from build123d import *

# Parameters (mm, degrees)
F0_R     = 49.7765250683
F1_DEPTH = 152.4
F2_R     = 25.4
F4_D     = 76.2


# Not quite as in the source:
# - the program builds the solid bodies; features that only make, move or delete a surface that nothing else refers to are left out


with BuildPart() as f1:
    # F0 (on Top) → F1 (new body)
    with BuildSketch(Plane.XY):
        Circle(F0_R)
    extrude(amount=F1_DEPTH)

    # F2
    f2_edges = [f1.edges().sort_by_distance(p)[0] for p in [
        (-49.776525, 0, 152.4),
    ]]
    fillet(f2_edges, radius=F2_R)

    # F4 (through all)
    with Locations(Plane.XY.offset(152.4)):
        with Locations((0, 0)):
            Hole(F4_D / 2)


solid = f1.part
For this review, take the finished solid that the model builds, in its own axes (mm). Give positions to 0.01 mm unless a question says otherwise; leave off trailing zeros. Order: outer loops, then holes, each group sorted by start corner. A loop starts at its lowest first (then second) coordinate and runs counter-clockwise, first axis right, second up. Notation, with made-up numbers: M -32,-3 L 18,-3 A16 ccw 18,24 Z; hole C 70,72 d6. An arc over 180 degrees is marked long. Answer in a Markdown table with one row per item. Add a question column.
(1) Mouldability with a two-part tool opening along Y and no side actions: class faces 1 (the face through (-11, -37, 0)), 2 (the face through (22.97, -44.16, 62.61)), 3 (the face through (30.235, -23.183, 73.148)) as +Y half, -Y half, draft (parallel to the pull), parting line (faces both ways), or undercut.
(2) Wall thickness on probe 1 along Y at (x, z) = (0, 99.5); probe 2 along X at (y, z) = (-1.5, 110); probe 3 along Y at (x, z) = (35, 86.5): over which ranges is each line inside the solid? List them lowest first. Write a range as [from, to].
(3) For pin 1 (10 mm diameter, centred on x = 34, z = 94.5, fed in from +Y); pin 2 (1.5 mm diameter, centred on x = 2, z = 106.5, fed in from +Y); pin 3 (12 mm diameter, centred on x = -28.5, z = 131.5, fed in from +Y), all flat-tipped, find the tip position at first contact; note any pin that passes through.
(4) Consider section A-A on z = 96. State the section outline as (x, y) points, and give its area (3 significant figures).
Evaluation:
| question | item | result |
|---|---|---|
| 1 | face 1 | draft |
| 1 | face 2 | parting line |
| 1 | face 3 | undercut |
| 2 | probe 1 | y = [-49.78, -38.1], [38.1, 49.78] |
| 2 | probe 2 | x = [-49.75, -38.07], [38.07, 49.75] |
| 2 | probe 3 | y = [-35.39, -15.05], [15.05, 35.39] |
| 3 | pin 1 | stops at y = 40.46 |
| 3 | pin 2 | stops at y = 49.76 |
| 3 | pin 3 | stops at y = 44.1 |
| 4 | outline | C 0,0 d99.55; hole C 0,0 d76.2 |
| 4 | area | 3,220 mm^2 |
